```python
from build123d import *

# Parameters (mm, degrees)
SKETCH1_R           = 7
BOSS_EXTRUDE1_DEPTH = 48
SKETCH2_R           = 5.8
CUT_EXTRUDE1_DEPTH  = 0.1
SKETCH3_R           = 5.25
CUT_EXTRUDE2_DEPTH  = 0.1
SKETCH4_R           = 5.05
SKETCH4_R_2         = 3.45
BOSS_EXTRUDE2_DEPTH = 0.1
FILLET1_R           = 0.5
SKETCH5_R           = 3.35
BOSS_EXTRUDE3_DEPTH = 0.1
BOSS_EXTRUDE3_TAPER = 46
FILLET4_R           = 0.1
SKETCH6_R           = 4.39
BOSS_EXTRUDE4_DEPTH = 0.15
BOSS_EXTRUDE4_TAPER = 74
SKETCH7_R           = 2.7
BOSS_EXTRUDE5_DEPTH = 1.4
BOSS_EXTRUDE5_TAPER = 5
FILLET5_R           = 0.5
FILLET6_R           = 0.5


with BuildPart() as part:
    # Sketch1 → Boss-Extrude1 (new body)
    with BuildSketch(Plane(origin=(0, 0, 0), x_dir=(0, 0, -1), z_dir=(1, 0, 0))):
        Circle(SKETCH1_R)
    extrude(amount=BOSS_EXTRUDE1_DEPTH)

    # Sketch2 → Cut-Extrude1 (cut)
    with BuildSketch(Plane(origin=(48, 0, 0), x_dir=(0, 0, -1), z_dir=(1, 0, 0))):
        Circle(SKETCH2_R)
    extrude(amount=-CUT_EXTRUDE1_DEPTH, mode=Mode.SUBTRACT)

    # Sketch3 → Cut-Extrude2 (cut)
    with BuildSketch(Plane.ZY):
        Circle(SKETCH3_R)
    extrude(amount=-CUT_EXTRUDE2_DEPTH, mode=Mode.SUBTRACT)

    # Sketch4 → Boss-Extrude2 (add)
    with BuildSketch(Plane.ZY.offset(-0.1)):
        Circle(SKETCH4_R)
        Circle(SKETCH4_R_2, mode=Mode.SUBTRACT)
    extrude(amount=BOSS_EXTRUDE2_DEPTH)

    # Fillet1
    # the kernel refuses this fillet: 0.5 mm, written as the material it takes off along each edge
    with BuildSketch(Plane(origin=(0, 0, 0), x_dir=(0, 0, 1), z_dir=(0, -1, 0))) as fillet1_piece_1:
        with BuildLine():
            CenterArc((4.75, -0.5), FILLET1_R, 53.130102354, 36.869897646)
            Line((4.75, 0), (4.75, 0.01))
            Line((4.75, 0.01), (5.05, 0.01))
            Line((5.05, 0.01), (5.06, 0))
            ThreePointArc((5.06, 0), (5.06, -0.05), (5.056, -0.092))
            Line((5.056, -0.092), (5.05, -0.1))
        make_face()
    revolve(axis=Axis((0, 0, 0), (-1, 0, 0)), mode=Mode.SUBTRACT)
    with BuildSketch(Plane(origin=(0, 0, 0), x_dir=(0, 0, 1), z_dir=(0, -1, 0))) as fillet1_piece_2:
        with BuildLine():
            CenterArc((3.75, -0.5), FILLET1_R, 90, 36.869897646)
            Line((3.45, -0.1), (3.444, -0.092))
            ThreePointArc((3.444, -0.092), (3.44, -0.05), (3.44, 0))
            Line((3.44, 0), (3.45, 0.01))
            Line((3.45, 0.01), (3.75, 0.01))
            Line((3.75, 0.01), (3.75, 0))
        make_face()
    revolve(axis=Axis((0, 0, 0), (-1, 0, 0)), mode=Mode.SUBTRACT)

    # Sketch5 → Boss-Extrude3 (add)
    with BuildSketch(Plane.ZY.offset(-0.1)):
        Circle(SKETCH5_R)
    extrude(amount=BOSS_EXTRUDE3_DEPTH, taper=BOSS_EXTRUDE3_TAPER)

    # Fillet4
    fillet4_edges = [part.edges().sort_by_distance(p)[0] for p in [
        (0.1, 0, -3.45),
        (0.1, 0, -3.35),
        (0, 0, -3.246446969),
    ]]
    fillet(fillet4_edges, radius=FILLET4_R)

    # Sketch6 → Boss-Extrude4 (add)
    with BuildSketch(Plane(origin=(47.9, 0, 0), x_dir=(0, 0, -1), z_dir=(1, 0, 0))):
        Circle(SKETCH6_R)
    extrude(amount=BOSS_EXTRUDE4_DEPTH, taper=BOSS_EXTRUDE4_TAPER)

    # Sketch7 → Boss-Extrude5 (add)
    with BuildSketch(Plane(origin=(48.05, 0, 0), x_dir=(0, 0, -1), z_dir=(1, 0, 0))):
        Circle(SKETCH7_R)
    extrude(amount=BOSS_EXTRUDE5_DEPTH, taper=BOSS_EXTRUDE5_TAPER)

    # Fillet5
    fillet5_edges = [part.edges().sort_by_distance(p)[0] for p in [
        (48.05, 0, 2.7),
    ]]
    fillet(fillet5_edges, radius=FILLET5_R)

    # Fillet6
    fillet6_edges = [part.edges().sort_by_distance(p)[0] for p in [
        (49.45, 0, 2.577515871),
    ]]
    fillet(fillet6_edges, radius=FILLET6_R)


solid = part.part
```
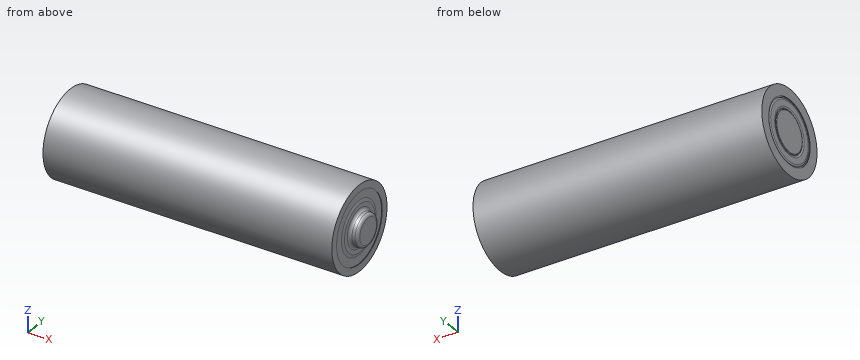
Check sheet for the modelled part. Datum: model origin and axes. Units: mm. Coordinates: 2 decimals unless noted, no trailing zeros. Order: outer loops, then holes, each group sorted by start corner. A loop starts at its lowest first (then second) coordinate and runs counter-clockwise, first axis right, second up. Notation, with made-up numbers: M 44,40 L 103,40 A34 cw 103,73 Z; hole C 55.25,2 d9. An arc over 180 degrees is marked long. One line per question, with ' | ' between items. Start each with the question number.
Item 1: Gauge pin test, flat ends, axial feed: P1, Ø1.5, axis at x = 36, z = 2, coming from the +Y side; P2, Ø2, axis at x = 25.5, y = 4.5, coming from the -Z side; P3, Ø3, axis at x = 13.5, z = 3, coming from the +Y side. Record the tip position at first contact, or that the pin passes through.
Item 2: Material ranges on line 1 (X direction, y = -3.75, z = 4); line 2 (X direction, y = -3.25, z = 5.25); line 3 (Z direction, x = 35, y = -0.25), recorded low to high.
Item 3: Sectioned sample at A-A on x = 7.5. Record the cut outline in (y, z).
Answer below:
1) P1: stops at y = 6.89 | P2: stops at z = -6.06 | P3: stops at y = 6.84
2) line 1: x = 0 to 47.9 | line 2: x = 0 to 48 | line 3: z = -7 to 7
3) outline: C 0,0 d14
